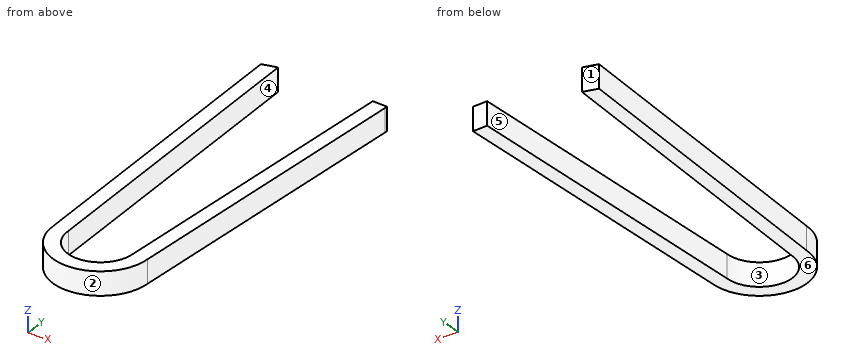
```python
from build123d import *

# Parameters (mm, degrees)
F1_DEPTH = 5.588


with BuildPart() as f1:
    # F0 (on Top) → F1 (new body)
    with BuildSketch(Plane.XY):
        with BuildLine():
            Line((-14.997657, 75.743783), (-11.388115, 0))
            ThreePointArc((-11.388115, 0), (0, -11.388115), (11.388115, 0))
            Line((11.388115, 0), (14.997657, 75.743783))
            Line((14.997657, 75.743783), (15.031717, 76.458491))
            Line((15.031717, 76.458491), (11.479748, 76.627759))
            Line((11.479748, 76.627759), (7.831738, 0.076784))
            ThreePointArc((7.831738, 0.076784), (0, -7.832115), (-7.831738, 0.076784))
            Line((-7.831738, 0.076784), (-11.479748, 76.627759))
            Line((-11.479748, 76.627759), (-14.997657, 75.743783))
        make_face()
    extrude(amount=F1_DEPTH)


solid = f1.part
```
Input: part model. Units: mm. Frame: model coordinates. Face numbers are marked on the shaded views. A direction names the side the tool comes from. Round coordinates to 2 decimals unless told otherwise and drop trailing zeros. Loops run counter-clockwise (first coordinate to the right, second up) from the corner with the lowest first, then second, coordinate; pieces in that order, holes last. Notation, with made-up numbers: (58, -19) - (73, -19) arc R10 cw to (73, -14) - close; hole circle Ø2 at (33.5, 66). An arc over 180 degrees is marked (long way). One line per item, written item: value. Start each with the question number.
(1) Draft query along X for the marked faces 1, 2, 3 and 4. Return one class per face: +X half, -X half, draft (parallel to the pull), parting line (faces both ways), or undercut.
(2) Section C-C, the plane x = -13. Return loops of the section in (y, z).
(3) Contact query for flat-ended pins moving along their axis: P1, Ø2, axis at y = 60.5, z = 3.5, coming from the -X side; P2, Ø1.5, axis at y = 63.5, z = 1.5, coming from the +X side; P3, Ø8, axis at x = 5.5, y = 12.5, coming from the -Z side; P4, Ø3, axis at y = 67, z = 3.5, coming from the -X side. Output: stop coordinate, or through.
(4) Ray query, line 1 (X direction, y = 41, z = 1.1); line 2 (X direction, y = 29.5, z = 0.5); line 3 (Y direction, x = 3, z = 1.2). Return the intervals inside material, ascending. Write a range as [from, to].
(5) Access query for the marked faces 5 and 6. Directions: +Z, -Z, +X, -X, +Y, -Y. A direction counts if a zero-diameter tool reaches every point of the face in a straight line with its end or side. Return the directions, or none.
(6) Section B-B, the plane x = 0. Return loops of the section in (y, z).
(7) Section A-A, the plane y = 52.5. Return loops of the section in (x, z), plus the area to 3 significant figures.
Results below:
1. face 1: -X half
1. face 2: parting line
1. face 3: undercut
1. face 4: undercut
2. outline: (33.82, 0) - (76.25, 0) - (76.25, 5.59) - (33.82, 5.59) - close
3. P1: x = -14.32
3. P2: x = 14.45
3. P3: z = 0
3. P4: x = -14.65
4. line 1: [-13.34, -9.78], [9.78, 13.34]
4. line 2: [-12.79, -9.23], [9.23, 12.79]
4. line 3: [-10.99, -7.23]
5. face 5: +Z, -Z, +Y
5. face 6: -Z, +X, -X, +Y, -Y
6. outline: (-11.39, 0) - (-7.83, 0) - (-7.83, 5.59) - (-11.39, 5.59) - close
7. outline: (-13.89, 0) - (-10.33, 0) - (-10.33, 5.59) - (-13.89, 5.59) - close; (10.33, 0) - (13.89, 0) - (13.89, 5.59) - (10.33, 5.59) - close
7. area: 39.8 mm^2
